Verification items for the finished model (mm, model axes). Give positions to 0.01 mm unless a question says otherwise; leave off trailing zeros. Write each loop counter-clockwise with the first axis right and the second up, starting at its lowest first coordinate (ties: lowest second). Pieces come first, ordered by that corner, then holes.
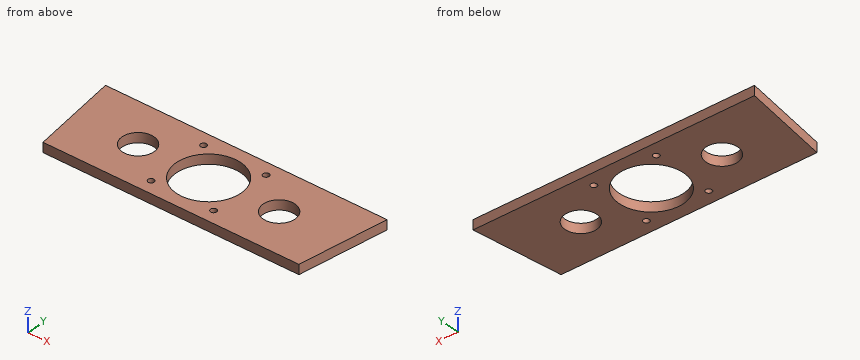
from build123d import *

# Parameters (mm, degrees)
BOSS_EXTRUDE1_DEPTH = 4.7625
SKETCH2_3_R         = 1.5
SKETCH2_3_R_2       = 7.874
SKETCH2_3_R_3       = 16
BOSS_EXTRUDE2_DEPTH = 4.7625
CUT_EXTRUDE1_DEPTH  = 4.7625


with BuildPart() as part:
    # Sketch2 → Boss-Extrude1 (new body)
    with BuildSketch(Plane.XY):
        Polygon((139.7, 6.35), (146.05, 50.8), (152.4, 50.8), (152.4, 0), (0, 0), (0, 50.8), (6.35, 50.8), (12.7, 6.35), align=None)
    extrude(amount=BOSS_EXTRUDE1_DEPTH)

    # Sketch2<3> → Boss-Extrude2 (add)
    # profile 1 of 2: a face of its own
    with BuildSketch(Plane.XY):
        Polygon((0, 50.8), (0, 0), (152.4, 0), (152.4, 50.8), (146.05, 50.8), (139.7, 6.35), (12.7, 6.35), (6.35, 50.8), align=None)
    # profile 2 of 2: a face of its own
    with BuildSketch(Plane.XY):
        Polygon((146.05, 50.8), (6.35, 50.8), (12.7, 6.35), (139.7, 6.35), align=None)
        with Locations((60.7, 13.075)):
            Circle(SKETCH2_3_R, mode=Mode.SUBTRACT)
        with Locations((91.7, 13.075)):
            Circle(SKETCH2_3_R, mode=Mode.SUBTRACT)
        with Locations((41.2, 28.575)):
            Circle(SKETCH2_3_R_2, mode=Mode.SUBTRACT)
        with Locations((60.7, 44.075)):
            Circle(SKETCH2_3_R, mode=Mode.SUBTRACT)
        with Locations((76.2, 28.575)):
            Circle(SKETCH2_3_R_3, mode=Mode.SUBTRACT)
        with Locations((111.2, 28.575)):
            Circle(SKETCH2_3_R_2, mode=Mode.SUBTRACT)
        with Locations((91.7, 44.075)):
            Circle(SKETCH2_3_R, mode=Mode.SUBTRACT)
    extrude(amount=BOSS_EXTRUDE2_DEPTH)

    # Sketch2<4> → Cut-Extrude1 (cut)
    with BuildSketch(Plane.XY):
        Polygon((139.7, 6.35), (146.05, 50.8), (152.4, 50.8), (152.4, 0), (0, 0), (0, 50.8), (6.35, 50.8), (12.7, 6.35), align=None)
    extrude(amount=CUT_EXTRUDE1_DEPTH, mode=Mode.SUBTRACT)


solid = part.part
Item 1: Sectioned sample at B-B on y = 40.5. Record the cut outline in (x, z), then the cut area to 3 significant figures.
Answer key:
outline: (7.82, 0) - (65.53, 0) - (65.53, 4.76) - (7.82, 4.76) - close; (86.87, 0) - (144.58, 0) - (144.58, 4.76) - (86.87, 4.76) - close
area: 550 mm2
Item 2: Sectioned sample at C-C on y = 26. Record the cut outline in (x, z).
Answer key:
outline: (9.89, 0) - (33.76, 0) - (33.76, 4.76) - (9.89, 4.76) - close; (48.64, 0) - (60.41, 0) - (60.41, 4.76) - (48.64, 4.76) - close; (91.99, 0) - (103.76, 0) - (103.76, 4.76) - (91.99, 4.76) - close; (118.64, 0) - (142.51, 0) - (142.51, 4.76) - (118.64, 4.76) - close
Item 3: Scan lines: line 1 along X through (y, z) = (29.5, 3.7); line 2 along X through (y, z) = (25, 0.2); line 3 along Y through (x, z) = (111.2, 3.05). Record each from-to range of solid material in increasing order.
Answer key:
line 1: x = 9.39 to 33.38, 49.02 to 60.23, 92.17 to 103.38, 119.02 to 143.01
line 2: x = 10.04 to 34.18, 48.22 to 60.6, 91.8 to 104.18, 118.22 to 142.36
line 3: y = 6.35 to 20.7, 36.45 to 50.8
Item 4: Depth check by flat-ended pin: pin 1 (1.8 mm diameter, centred on x = 60.7, y = 13.075, fed in from -Z); pin 2 (2 mm diameter, centred on y = 30.5, z = 2.5, fed in from -X). Enter the tip coordinate at first touch or a pass-through.
Answer key:
pin 1: passes through
pin 2: stops at x = 9.11
